from build123d import *

# Parameters (mm, degrees)
SKETCH2_R          = 6.5
SKETCH2_R_2        = 4.5
CUT_EXTRUDE1_DEPTH = 0.5


with BuildPart() as part:
    # Sketch1 → Revolve1 (revolve)
    with BuildSketch(Plane.XY, mode=Mode.PRIVATE) as revolve1_sk:
        Polygon((4, -12), (4, 12), (7, 12), (7.5, 11.5), (7.5, 8.75), (7, 8.75), (7, 7.65), (7.5, 7.65), (7.5, -7.65), (7, -7.65), (7, -8.75), (7.5, -8.75), (7.5, -11.5), (7, -12), align=None)
    revolve(revolve1_sk.sketch.rotate(Axis((0, 12, 0), (0, -1, 0)), 180), axis=Axis((0, 12, 0), (0, -1, 0)))

    # Sketch2 → Cut-Extrude1 (cut)
    with BuildSketch(Plane(origin=(0, 12, 0), x_dir=(1, 0, 0), z_dir=(0, 1, 0))):
        with Locations(Location((0, 0, 0), (0, 0, 180))):
            Circle(SKETCH2_R)
        with Locations(Location((0, 0, 0), (0, 0, 180))):
            Circle(SKETCH2_R_2, mode=Mode.SUBTRACT)
    cut_extrude1 = extrude(amount=-CUT_EXTRUDE1_DEPTH, mode=Mode.SUBTRACT)

    # Mirror1: Cut-Extrude1 across plane
    add(cut_extrude1.mirror(Plane.ZX), mode=Mode.SUBTRACT)


solid = part.part
CAD build for the part. Positions are in the model's coordinates, mm. A direction names the side the tool comes from. Round coordinates to 2 decimals unless told otherwise and drop trailing zeros. Loops run counter-clockwise (first coordinate to the right, second up) from the corner with the lowest first, then second, coordinate; pieces in that order, holes last. Notation, with made-up numbers: (-32, 79) - (-11, 79) arc R35 cw to (-11, 112) - close; hole circle Ø8 at (28.25, 81). An arc over 180 degrees is marked (long way). Put each result on its own line as item: value.
1. Pin check, flat tips, straight feed: P1, Ø1.5, axis at y = -6.5, z = 5.5, coming from the -X side; P2, Ø3, axis at x = 5, y = 3.5, coming from the +Z side; P3, Ø5, axis at x = -5.5, y = -7.5, coming from the +Z side. Stop position of each tip, or through.
Geometry check:
P1: x = -5.8
P2: z = 6.63
P3: z = 6.87
2. Wall check: line 1 (Z direction, x = 2.5, y = 3.25); line 2 (Y direction, x = -5.5, z = 4.75); line 3 (Z direction, x = -3.25, y = 7). Give the ranges that are in metal, low to high.
Geometry check:
line 1: -7.07 to -3.12, 3.12 to 7.07
line 2: -11.73 to -8.75, -7.65 to 7.65, 8.75 to 11.73
line 3: -6.76 to -2.33, 2.33 to 6.76
3. Two-plate mould, pull along X, no slides. Class faces 1 (the flat face through (-2, 7.65, 7)), 2 (the cylindrical face through (-6.466, 8.192, 2.681)), 3 (the flat face through (1.54, 11.5, 4.42)): released by +X, released by -X, zero draft, split by the parting line, or undercut.
Geometry check:
face 1: zero draft
face 2: split by the parting line
face 3: undercut
4. Slice it at A-A on y = -8. List the corners of the cut face in (x, z), and give its area (3 significant figures).
Geometry check:
outline: circle Ø14 at (0, 0); hole circle Ø8 at (0, 0)
area: 104 mm²
5. 3-axis set-ups, long thin cutter, end or side, ignore diameter. For faces 4 (the cylindrical face through (3.32, 11.75, 3.04)), 5 (the flat face through (2, -7.65, 7)), 6 (the flat face through (3, -12, 3)), 7 (the cylindrical face through (0.867, 0.168, 3.905)), 8 (the cylindrical face through (5.158, -11.754, -3.955)): which of +Z, -Z, +X, -X, +Y, -Y reach the whole face in a straight line?
Geometry check:
face 4: +Y
face 5: none
face 6: +Z, -Z, +X, -X, -Y
face 7: +Y, -Y
face 8: -Y
